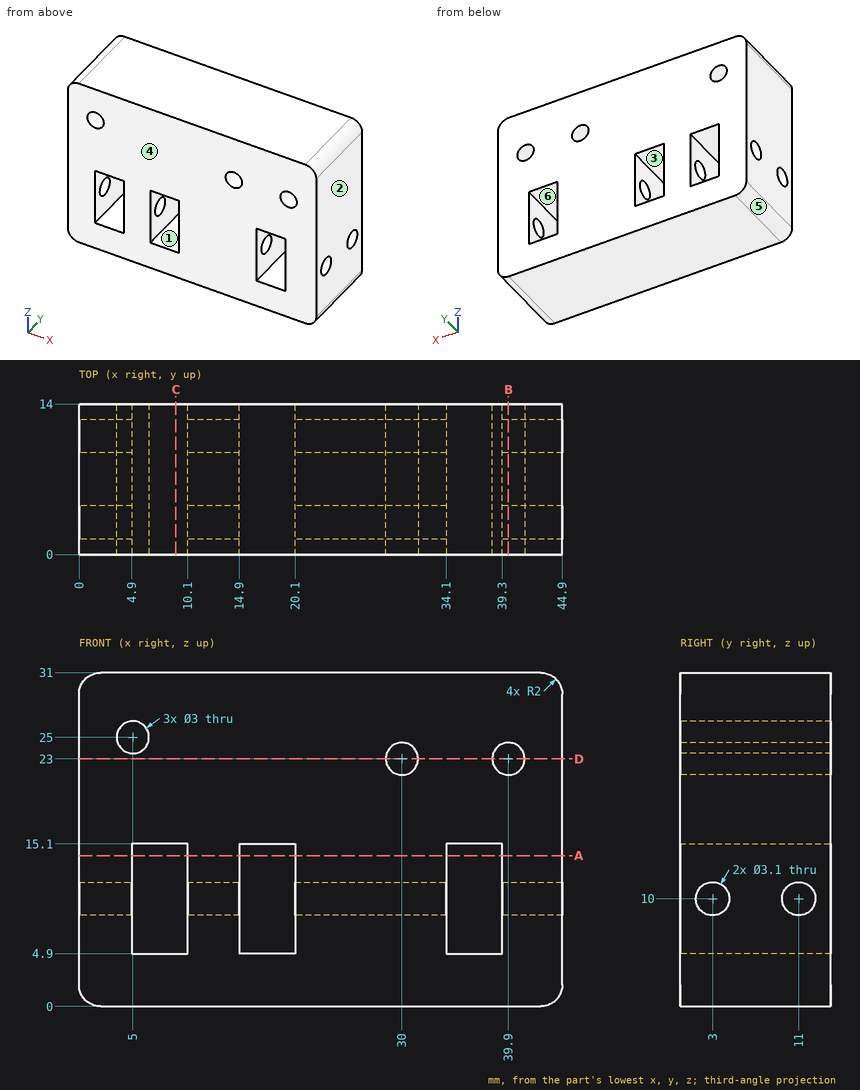
Geometry check sheet. Reference: drawing and pictorial views, mm from the part's lowest x, y, z. A direction names the side the tool comes from. Coordinates: 2 decimals unless noted, no trailing zeros. Order: outer loops, then holes, each group sorted by start corner. A loop starts at its lowest first (then second) coordinate and runs counter-clockwise, first axis right, second up. Notation, with made-up numbers: (35.25, -8.75) -> (49.25, -8.75) arc R22 cw to (49.25, 21.25) -> close; hole circle Ø7 at (26, -29.5). An arc over 180 degrees is marked (long way). Put each result on its own line as item: value. Start each with the question number.
1) Release check for a two-part mould opening along X. For the marked faces 3, 4, 5 and 6 record: pulls with the +X half, pulls with the -X half, needs draft (parallel to the pull), parting line crosses it, or undercut.
2) Material ranges on L1, parallel to Y at x = 11, z = 10; L2, parallel to X at y = 5, z = 6.5; L3, parallel to Z at x = 15, y = 8.5, recorded low to high.
3) Tool access check on the marked faces 1 and 2. Record the directions out of +Z, -Z, +X, -X, +Y, -Y that give a thin tool (end or side, any length) a straight path to the whole face; none if there is none.
4) Cross-section at B-B (x = 39.9). Enter the section's corners in (y, z).
5) Cross-section at A-A (z = 14). Enter the section's corners in (x, y).
6) Go/stop test with a flat-tipped pin: pin 1 (1.9 mm diameter, centred on y = 3, z = 10, fed in from -X) (3 decimals). Record where the tip stops, or that it passes through.
7) Cross-section at D-D (z = 23). Enter the section's corners in (x, y), plus the area to 3 significant figures.
8) Cross-section at C-C (x = 9). Enter the section's corners in (y, z).
Geometry check:
1. face 3: undercut
1. face 4: needs draft
1. face 5: pulls with the -X half
1. face 6: undercut
2. L1: y = 0 to 1.45, 4.55 to 9.45, 12.55 to 14
2. L2: x = 0 to 4.9, 10.1 to 14.9, 20.1 to 34.1, 39.3 to 44.9
2. L3: z = 0 to 4.9, 15.1 to 31
3. face 1: +Y, -Y
3. face 2: +Z, -Z, +X, +Y, -Y
4. outline: (0, 0) -> (14, 0) -> (14, 21.5) -> (0, 21.5) -> close; (0, 24.5) -> (14, 24.5) -> (14, 31) -> (0, 31) -> close; hole circle Ø3.1 at (3, 10); hole circle Ø3.1 at (11, 10)
5. outline: (0, 0) -> (4.9, 0) -> (4.9, 14) -> (0, 14) -> close; (10.1, 0) -> (14.9, 0) -> (14.9, 14) -> (10.1, 14) -> close; (20.1, 0) -> (34.1, 0) -> (34.1, 14) -> (20.1, 14) -> close; (39.3, 0) -> (44.9, 0) -> (44.9, 14) -> (39.3, 14) -> close
6. pin 1: passes through
7. outline: (0, 0) -> (28.5, 0) -> (28.5, 14) -> (0, 14) -> close; (31.5, 0) -> (38.4, 0) -> (38.4, 14) -> (31.5, 14) -> close; (41.4, 0) -> (44.9, 0) -> (44.9, 14) -> (41.4, 14) -> close
7. area: 545 mm^2
8. outline: (0, 0) -> (14, 0) -> (14, 4.9) -> (0, 4.9) -> close; (0, 15.1) -> (14, 15.1) -> (14, 31) -> (0, 31) -> close
